Geometry: final body of the model. Coordinates: model frame, mm. Give positions to 0.01 mm unless a question says otherwise; leave off trailing zeros. Write each loop counter-clockwise with the first axis right and the second up, starting at its lowest first coordinate (ties: lowest second). Pieces come first, ordered by that corner, then holes.
Q1. Cut plane A-A on y = -4.5. Return the cut outline in (x, z), plus the area to 3 significant figures.
Q2. Line query: L1, parallel to X at y = 6.75, z = 20.5; L2, parallel to Y at x = 2.5, z = 89.5; L3, parallel to X at y = -15.5, z = 44.5. Output: solid intervals per line, ascending.
Q3. Cut plane B-B on x = -6. Return the cut outline in (y, z), plus the area to 3 significant figures.
Q4. Cut plane C-C on z = 67. Count the separate pieces of the cut face and the enclosed holes in it, plus the area to 3 significant figures.
Q5. Pin query (flat end, axial travel): pin 1 (7 mm diameter, centred on x = -8, z = 58.5, fed in from -Y); pin 2 (0.6 mm diameter, centred on y = -10, z = 68, fed in from +X); pin 3 (4 mm diameter, centred on x = -9.5, z = 33.5, fed in from +Y). Return the tip coordinate at first contact, or that it passes through.
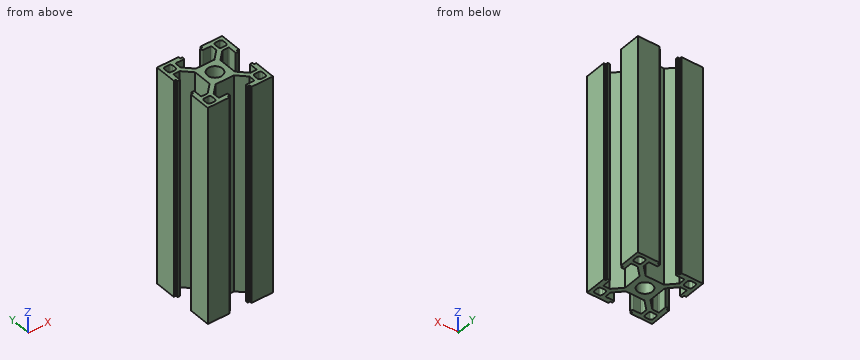
```python
from build123d import *

# Parameters (mm, degrees)
SKETCH_1_R      = 3.4
EXTRUDE_1_DEPTH = 100


with BuildPart() as part:
    # 草图1 → 凸台-拉伸1 (new body)
    with BuildSketch(Plane.XY):
        with BuildLine():
            Line((-23.424024871, 7.005983494), (-23.424024871, -0.394016506))
            Line((-23.424024871, -0.394016506), (-22.624024871, -0.394016506))
            ThreePointArc((-22.624024871, -0.394016506), (-22.482603515, -0.45259515), (-22.424024871, -0.594016506))
            Line((-22.424024871, -0.594016506), (-22.424024871, -1.394016506))
            Line((-22.424024871, -1.394016506), (-21.524024871, -1.394016506))
            ThreePointArc((-21.524024871, -1.394016506), (-21.311892836, -1.306148541), (-21.224024871, -1.094016506))
            Line((-21.224024871, -1.094016506), (-21.224024871, 2.455983494))
            ThreePointArc((-21.224024871, 2.455983494), (-21.136156905, 2.668115528), (-20.924024871, 2.755983494))
            Line((-20.924024871, 2.755983494), (-18.229659789, 2.755983494))
            Line((-18.229659789, 2.755983494), (-14.224024871, -1.249651425))
            Line((-14.224024871, -1.249651425), (-14.224024871, -9.738381588))
            Line((-14.224024871, -9.738381588), (-18.229659789, -13.744016506))
            Line((-18.229659789, -13.744016506), (-20.924024871, -13.744016506))
            ThreePointArc((-20.924024871, -13.744016506), (-21.136156905, -13.656148541), (-21.224024871, -13.444016506))
            Line((-21.224024871, -13.444016506), (-21.224024871, -9.894016506))
            ThreePointArc((-21.224024871, -9.894016506), (-21.311892836, -9.681884472), (-21.524024871, -9.594016506))
            Line((-21.524024871, -9.594016506), (-22.424024871, -9.594016506))
            Line((-22.424024871, -9.594016506), (-22.424024871, -10.394016506))
            ThreePointArc((-22.424024871, -10.394016506), (-22.482603515, -10.535437862), (-22.624024871, -10.594016506))
            Line((-22.624024871, -10.594016506), (-23.424024871, -10.594016506))
            Line((-23.424024871, -10.594016506), (-23.424024871, -17.994016506))
            Line((-23.424024871, -17.994016506), (-23.424024871, -20.494016506))
            Line((-23.424024871, -20.494016506), (-20.924024871, -20.494016506))
            Line((-20.924024871, -20.494016506), (-13.524024871, -20.494016506))
            Line((-13.524024871, -20.494016506), (-13.524024871, -19.694016506))
            ThreePointArc((-13.524024871, -19.694016506), (-13.465446227, -19.55259515), (-13.324024871, -19.494016506))
            Line((-13.324024871, -19.494016506), (-12.524024871, -19.494016506))
            Line((-12.524024871, -19.494016506), (-12.524024871, -18.594016506))
            ThreePointArc((-12.524024871, -18.594016506), (-12.611892836, -18.381884472), (-12.824024871, -18.294016506))
            Line((-12.824024871, -18.294016506), (-16.374024871, -18.294016506))
            ThreePointArc((-16.374024871, -18.294016506), (-16.586156905, -18.206148541), (-16.674024871, -17.994016506))
            Line((-16.674024871, -17.994016506), (-16.674024871, -15.299651425))
            Line((-16.674024871, -15.299651425), (-12.668389952, -11.294016506))
            Line((-12.668389952, -11.294016506), (-4.179659789, -11.294016506))
            Line((-4.179659789, -11.294016506), (-0.174024871, -15.299651425))
            Line((-0.174024871, -15.299651425), (-0.174024871, -17.994016506))
            ThreePointArc((-0.174024871, -17.994016506), (-0.261892836, -18.206148541), (-0.474024871, -18.294016506))
            Line((-0.474024871, -18.294016506), (-4.024024871, -18.294016506))
            ThreePointArc((-4.024024871, -18.294016506), (-4.236156905, -18.381884472), (-4.324024871, -18.594016506))
            Line((-4.324024871, -18.594016506), (-4.324024871, -19.494016506))
            Line((-4.324024871, -19.494016506), (-3.524024871, -19.494016506))
            ThreePointArc((-3.524024871, -19.494016506), (-3.382603515, -19.55259515), (-3.324024871, -19.694016506))
            Line((-3.324024871, -19.694016506), (-3.324024871, -20.494016506))
            Line((-3.324024871, -20.494016506), (4.075975129, -20.494016506))
            Line((4.075975129, -20.494016506), (6.575975129, -20.494016506))
            Line((6.575975129, -20.494016506), (6.575975129, -17.994016506))
            Line((6.575975129, -17.994016506), (6.575975129, -10.594016506))
            Line((6.575975129, -10.594016506), (5.775975129, -10.594016506))
            ThreePointArc((5.775975129, -10.594016506), (5.634553773, -10.535437862), (5.575975129, -10.394016506))
            Line((5.575975129, -10.394016506), (5.575975129, -9.594016506))
            Line((5.575975129, -9.594016506), (4.675975129, -9.594016506))
            ThreePointArc((4.675975129, -9.594016506), (4.463843095, -9.681884472), (4.375975129, -9.894016506))
            Line((4.375975129, -9.894016506), (4.375975129, -13.444016506))
            ThreePointArc((4.375975129, -13.444016506), (4.288107164, -13.656148541), (4.075975129, -13.744016506))
            Line((4.075975129, -13.744016506), (1.381610048, -13.744016506))
            Line((1.381610048, -13.744016506), (-2.624024871, -9.738381588))
            Line((-2.624024871, -9.738381588), (-2.624024871, -1.249651425))
            Line((-2.624024871, -1.249651425), (1.381610048, 2.755983494))
            Line((1.381610048, 2.755983494), (4.075975129, 2.755983494))
            ThreePointArc((4.075975129, 2.755983494), (4.288107164, 2.668115528), (4.375975129, 2.455983494))
            Line((4.375975129, 2.455983494), (4.375975129, -1.094016506))
            ThreePointArc((4.375975129, -1.094016506), (4.463843095, -1.306148541), (4.675975129, -1.394016506))
            Line((4.675975129, -1.394016506), (5.575975129, -1.394016506))
            Line((5.575975129, -1.394016506), (5.575975129, -0.594016506))
            ThreePointArc((5.575975129, -0.594016506), (5.634553773, -0.45259515), (5.775975129, -0.394016506))
            Line((5.775975129, -0.394016506), (6.575975129, -0.394016506))
            Line((6.575975129, -0.394016506), (6.575975129, 7.005983494))
            Line((6.575975129, 7.005983494), (6.575975129, 9.505983494))
            Line((6.575975129, 9.505983494), (4.075975129, 9.505983494))
            Line((4.075975129, 9.505983494), (-3.324024871, 9.505983494))
            Line((-3.324024871, 9.505983494), (-3.324024871, 8.705983494))
            ThreePointArc((-3.324024871, 8.705983494), (-3.382603515, 8.564562138), (-3.524024871, 8.505983494))
            Line((-3.524024871, 8.505983494), (-4.324024871, 8.505983494))
            Line((-4.324024871, 8.505983494), (-4.324024871, 7.605983494))
            ThreePointArc((-4.324024871, 7.605983494), (-4.236156905, 7.393851459), (-4.024024871, 7.305983494))
            Line((-4.024024871, 7.305983494), (-0.474024871, 7.305983494))
            ThreePointArc((-0.474024871, 7.305983494), (-0.261892836, 7.218115528), (-0.174024871, 7.005983494))
            Line((-0.174024871, 7.005983494), (-0.174024871, 4.311618412))
            Line((-0.174024871, 4.311618412), (-4.179659789, 0.305983494))
            Line((-4.179659789, 0.305983494), (-12.668389952, 0.305983494))
            Line((-12.668389952, 0.305983494), (-16.674024871, 4.311618412))
            Line((-16.674024871, 4.311618412), (-16.674024871, 7.005983494))
            ThreePointArc((-16.674024871, 7.005983494), (-16.586156905, 7.218115528), (-16.374024871, 7.305983494))
            Line((-16.374024871, 7.305983494), (-12.824024871, 7.305983494))
            ThreePointArc((-12.824024871, 7.305983494), (-12.611892836, 7.393851459), (-12.524024871, 7.605983494))
            Line((-12.524024871, 7.605983494), (-12.524024871, 8.505983494))
            Line((-12.524024871, 8.505983494), (-13.324024871, 8.505983494))
            ThreePointArc((-13.324024871, 8.505983494), (-13.465446227, 8.564562138), (-13.524024871, 8.705983494))
            Line((-13.524024871, 8.705983494), (-13.524024871, 9.505983494))
            Line((-13.524024871, 9.505983494), (-20.924024871, 9.505983494))
            Line((-20.924024871, 9.505983494), (-23.424024871, 9.505983494))
            Line((-23.424024871, 9.505983494), (-23.424024871, 7.005983494))
        make_face()
        with Locations((-8.424024871, -5.494016506)):
            Circle(SKETCH_1_R, mode=Mode.SUBTRACT)
        with BuildLine():
            Line((2.325975129, -15.244016506), (4.075975129, -15.244016506))
            ThreePointArc((4.075975129, -15.244016506), (4.78308191, -15.536909725), (5.075975129, -16.244016506))
            Line((5.075975129, -16.244016506), (5.075975129, -17.994016506))
            ThreePointArc((5.075975129, -17.994016506), (4.78308191, -18.701123287), (4.075975129, -18.994016506))
            Line((4.075975129, -18.994016506), (2.325975129, -18.994016506))
            ThreePointArc((2.325975129, -18.994016506), (1.618868348, -18.701123287), (1.325975129, -17.994016506))
            Line((1.325975129, -17.994016506), (1.325975129, -16.244016506))
            ThreePointArc((1.325975129, -16.244016506), (1.618868348, -15.536909725), (2.325975129, -15.244016506))
        make_face(mode=Mode.SUBTRACT)
        with BuildLine():
            Line((1.325975129, 5.255983494), (1.325975129, 7.005983494))
            ThreePointArc((1.325975129, 7.005983494), (1.618868348, 7.713090275), (2.325975129, 8.005983494))
            Line((2.325975129, 8.005983494), (4.075975129, 8.005983494))
            ThreePointArc((4.075975129, 8.005983494), (4.78308191, 7.713090275), (5.075975129, 7.005983494))
            Line((5.075975129, 7.005983494), (5.075975129, 5.255983494))
            ThreePointArc((5.075975129, 5.255983494), (4.78308191, 4.548876713), (4.075975129, 4.255983494))
            Line((4.075975129, 4.255983494), (2.325975129, 4.255983494))
            ThreePointArc((2.325975129, 4.255983494), (1.618868348, 4.548876713), (1.325975129, 5.255983494))
        make_face(mode=Mode.SUBTRACT)
        with BuildLine():
            Line((-18.174024871, -16.244016506), (-18.174024871, -17.994016506))
            ThreePointArc((-18.174024871, -17.994016506), (-18.46691809, -18.701123287), (-19.174024871, -18.994016506))
            Line((-19.174024871, -18.994016506), (-20.924024871, -18.994016506))
            ThreePointArc((-20.924024871, -18.994016506), (-21.631131652, -18.701123287), (-21.924024871, -17.994016506))
            Line((-21.924024871, -17.994016506), (-21.924024871, -16.244016506))
            ThreePointArc((-21.924024871, -16.244016506), (-21.631131652, -15.536909725), (-20.924024871, -15.244016506))
            Line((-20.924024871, -15.244016506), (-19.174024871, -15.244016506))
            ThreePointArc((-19.174024871, -15.244016506), (-18.46691809, -15.536909725), (-18.174024871, -16.244016506))
        make_face(mode=Mode.SUBTRACT)
        with BuildLine():
            Line((-19.174024871, 4.255983494), (-20.924024871, 4.255983494))
            ThreePointArc((-20.924024871, 4.255983494), (-21.631131652, 4.548876713), (-21.924024871, 5.255983494))
            Line((-21.924024871, 5.255983494), (-21.924024871, 7.005983494))
            ThreePointArc((-21.924024871, 7.005983494), (-21.631131652, 7.713090275), (-20.924024871, 8.005983494))
            Line((-20.924024871, 8.005983494), (-19.174024871, 8.005983494))
            ThreePointArc((-19.174024871, 8.005983494), (-18.46691809, 7.713090275), (-18.174024871, 7.005983494))
            Line((-18.174024871, 7.005983494), (-18.174024871, 5.255983494))
            ThreePointArc((-18.174024871, 5.255983494), (-18.46691809, 4.548876713), (-19.174024871, 4.255983494))
        make_face(mode=Mode.SUBTRACT)
    extrude(amount=EXTRUDE_1_DEPTH)


solid = part.part
```
Data:
1. outline: (-14.22, 0) - (-11.68, 0) - (-11.68, 100) - (-14.22, 100) - close; (-5.17, 0) - (-2.62, 0) - (-2.62, 100) - (-5.17, 100) - close
1. area: 510 mm2
2. L1: x = -23.42 to -21.92, -18.17 to -16.67, -0.17 to 1.33, 5.08 to 6.58
2. L2: y = -20.49 to -18.99, -15.24 to -13.74, 2.76 to 4.26, 8.01 to 9.51
2. L3: x = -23.42 to -21.59, -18.51 to -16.67, -0.17 to 1.66, 4.74 to 6.58
3. outline: (-11.29, 0) - (-7.88, 0) - (-7.88, 100) - (-11.29, 100) - close; (-3.11, 0) - (0.31, 0) - (0.31, 100) - (-3.11, 100) - close
3. area: 683 mm2
4. separate pieces: 1
4. enclosed holes: 5
4. area: 333 mm2
5. pin 1: stops at y = -11.29
5. pin 2: stops at x = 5.58
5. pin 3: stops at y = 0.31
